```python
from build123d import *

# Parameters (mm, degrees)
AUFSATZ_LINEAR_AUSTRAGEN1_DEPTH = 30
SKIZZE2_R                       = 7
SCHNITT_LINEAR_AUSTRAGEN1_DEPTH = 20
SKIZZE5_W                       = 8.1
SKIZZE5_H                       = 30
AUFSATZ_LINEAR_AUSTRAGEN2_DEPTH = 3
FASE2_SIZE                      = 0.5
FASE1_SIZE                      = 1
VERRUNDUNG1_R                   = 5
VERRUNDUNG2_R                   = 10
SCHNITT_LINEAR_AUSTRAGEN2_REACH = 113.597
SKIZZE8_R                       = 2.5
SCHNITT_LINEAR_AUSTRAGEN3_DEPTH = 112.202517957


with BuildPart() as part:
    # Skizze1 → Aufsatz-Linear austragen1 (new body)
    with BuildSketch(Plane(origin=(0, 0, 0), x_dir=(1, 0, 0), z_dir=(0, 1, 0))):
        Polygon((-105, 0), (-105, -13), (-70, -13), (-70, 8), (70, 8), (70, -13), (105, -13), (105, 0), (105, 20), (-105, 20), align=None)
    extrude(amount=AUFSATZ_LINEAR_AUSTRAGEN1_DEPTH)

    # Skizze2 → Schnitt-Linear austragen1 (cut)
    with BuildSketch(Plane(origin=(0, 30, 0), x_dir=(1, 0, 0), z_dir=(0, 1, 0))):
        with Locations(Location((-87.5, 0, 0), (0, 0, 270))):
            Circle(SKIZZE2_R)
        with Locations(Location((87.5, 0, 0), (0, 0, 270))):
            Circle(SKIZZE2_R)
    extrude(amount=-SCHNITT_LINEAR_AUSTRAGEN1_DEPTH, mode=Mode.SUBTRACT)

    # Skizze5 → Aufsatz-Linear austragen2 (add)
    with BuildSketch(Plane(origin=(0, 0, -20), x_dir=(-1, 0, 0), z_dir=(0, 0, -1))):
        with Locations((0, 15)):
            Rectangle(SKIZZE5_W, SKIZZE5_H)
    extrude(amount=AUFSATZ_LINEAR_AUSTRAGEN2_DEPTH)

    # Fase2
    fase2_edges = [part.edges().sort_by_distance(p)[0] for p in [
        (-4.05, 15, -23),
        (0, 0, -23),
        (4.05, 15, -23),
        (0, 30, -23),
    ]]
    chamfer(fase2_edges, length=FASE2_SIZE)

    # Fase1
    fase1_edges = [part.edges().sort_by_distance(p)[0] for p in [
        (-87.5, 30, -7),
        (87.5, 30, -7),
    ]]
    chamfer(fase1_edges, length=FASE1_SIZE)

    # Verrundung1
    verrundung1_edges = [part.edges().sort_by_distance(p)[0] for p in [
        (-70, 15, 13),
        (-105, 15, 13),
        (105, 15, -20),
        (-105, 15, -20),
        (105, 15, 13),
        (70, 15, 13),
    ]]
    fillet(verrundung1_edges, radius=VERRUNDUNG1_R)

    # Verrundung2
    verrundung2_edges = [part.edges().sort_by_distance(p)[0] for p in [
        (70, 15, -8),
        (-70, 15, -8),
    ]]
    fillet(verrundung2_edges, radius=VERRUNDUNG2_R)

    # Skizze8 → Schnitt-Linear austragen2 (cut, up to next)
    with BuildSketch(Plane(origin=(0, 0, 0), x_dir=(1, 0, 0), z_dir=(0, 1, 0)), mode=Mode.PRIVATE) as schnitt_linear_austragen2_sk1:
        with Locations(Location((87.5, 0, 0), (0, 0, 90))):
            Circle(SKIZZE8_R)
    schnitt_linear_austragen2_tool1 = extrude(schnitt_linear_austragen2_sk1.sketch, amount=SCHNITT_LINEAR_AUSTRAGEN2_REACH, mode=Mode.PRIVATE) & part.part
    # Skizze8 → Schnitt-Linear austragen2 (cut, up to next)
    with BuildSketch(Plane(origin=(0, 0, 0), x_dir=(1, 0, 0), z_dir=(0, 1, 0)), mode=Mode.PRIVATE) as schnitt_linear_austragen2_sk2:
        with Locations(Location((-87.5, 0, 0), (0, 0, 90))):
            Circle(SKIZZE8_R)
    schnitt_linear_austragen2_tool2 = extrude(schnitt_linear_austragen2_sk2.sketch, amount=SCHNITT_LINEAR_AUSTRAGEN2_REACH, mode=Mode.PRIVATE) & part.part
    add(schnitt_linear_austragen2_tool1.solids().sort_by_distance((87.5, 0, 0))[0], mode=Mode.SUBTRACT)
    add(schnitt_linear_austragen2_tool2.solids().sort_by_distance((-87.5, 0, 0))[0], mode=Mode.SUBTRACT)

    # Skizze9 → Schnitt-Linear austragen3 (cut, through all)
    with BuildSketch(Plane.XY.offset(-8)):
        Polygon((0, 17.5), (-2.5, 15), (0, 12.5), (2.5, 15), align=None)
    extrude(amount=-SCHNITT_LINEAR_AUSTRAGEN3_DEPTH, mode=Mode.SUBTRACT)


solid = part.part
```
Geometry check sheet. Reference: the model listing, model coordinates, mm. A direction names the side the tool comes from. Give positions to 0.01 mm unless a question says otherwise; leave off trailing zeros. Write each loop counter-clockwise with the first axis right and the second up, starting at its lowest first coordinate (ties: lowest second). Pieces come first, ordered by that corner, then holes. Notation, with made-up numbers: (-22.5, -11) -> (10.5, -11) arc R27 cw to (10.5, 6) -> close; hole circle Ø4 at (76, -8). An arc over 180 degrees is marked (long way). One line per question, with ' | ' between items.
Item 1: Sectioned sample at C-C, the plane x = 32. Record the boundary of the cut face in (y, z).
Determined:
outline: (0, -20) -> (30, -20) -> (30, -8) -> (0, -8) -> close
Item 2: Scan lines: line 1 along X through (y, z) = (23, -3); line 2 along X through (y, z) = (4, 4); line 3 along X through (y, z) = (7.5, 0). Record each from-to range of solid material in increasing order.
Determined:
line 1: -105 to -93.82, -81.18 to -68.66, 68.66 to 81.18, 93.82 to 105 | line 2: -105 to -70, 70 to 105 | line 3: -105 to -90, -85 to -69.8, 69.8 to 85, 90 to 105
Item 3: Depth check by flat-ended pin: pin 1 (6 mm diameter, centred on y = 6, z = 9, fed in from +X); pin 2 (4 mm diameter, centred on x = 90.5, z = 0.5, fed in from +Y); pin 3 (9 mm diameter, centred on x = 19.5, y = 18, fed in from +Z); pin 4 (9 mm diameter, centred on x = 29, y = 11, fed in from -Z). Enter the tip coordinate at first touch or a pass-through.
Determined:
pin 1: x = 105 | pin 2: y = 10 | pin 3: z = -8 | pin 4: z = -20
Item 4: Sectioned sample at A-A, the plane x = 87.5. Record the boundary of the cut face in (y, z).
Determined:
outline: (0, -20) -> (30, -20) -> (30, -8) -> (29, -7) -> (10, -7) -> (10, -2.5) -> (0, -2.5) -> close; (0, 2.5) -> (10, 2.5) -> (10, 7) -> (29, 7) -> (30, 8) -> (30, 13) -> (0, 13) -> close
Item 5: Access from +Z, -Z, +X, -X, +Y, -Y to the whole of each face (thin tool, end or side, straight path). Record for faces 4 (the cylindrical face through (85, 5, 0)), 5 (the flat face through (-1, 11, -8)), 6 (the flat face through (-87, 10, 3)).
Determined:
face 4: +Y, -Y | face 5: +Z, +Y, -Y | face 6: +Y
Item 6: Sectioned sample at B-B, the plane z = 0. Record the boundary of the cut face in (x, y), plus the area to 3 significant figures.
Determined:
outline: (-105, 0) -> (-90, 0) -> (-90, 10) -> (-94.5, 10) -> (-94.5, 29) -> (-95.5, 30) -> (-105, 30) -> close; (-85, 0) -> (-69.8, 0) -> (-69.8, 30) -> (-79.5, 30) -> (-80.5, 29) -> (-80.5, 10) -> (-85, 10) -> close; (69.8, 0) -> (85, 0) -> (85, 10) -> (80.5, 10) -> (80.5, 29) -> (79.5, 30) -> (69.8, 30) -> close; (90, 0) -> (105, 0) -> (105, 30) -> (95.5, 30) -> (94.5, 29) -> (94.5, 10) -> (90, 10) -> close | area: 1,450 mm^2
Item 7: Draft check along Z on faces 1 (the cylindrical face through (-104, 15, 11)), 2 (the cylindrical face through (94.44, 19.63, -0.91)), 3 (the flat face through (-51, 15, -20)). Enter one of: released by +Z, released by -Z, zero draft, split by the parting line, or undercut.
Determined:
face 1: released by +Z | face 2: undercut | face 3: released by -Z
